Source: CAD feature listing. Evaluate the final solid. Frame: model axes, mm. A direction names the side the tool comes from. Coordinates: 2 decimals unless noted, no trailing zeros. Order: outer loops, then holes, each group sorted by start corner. A loop starts at its lowest first (then second) coordinate and runs counter-clockwise, first axis right, second up.
```python
from build123d import *

# Parameters (mm, degrees)
BOSS_EXTRUDE1_DEPTH = 15


with BuildPart() as part:
    # Sketch1 → Boss-Extrude1 (new body)
    with BuildSketch(Plane.XY):
        with BuildLine():
            Line((-3, 22.75), (-12, 16))
            ThreePointArc((-12, 16), (0, -20), (12, 16))
            Line((12, 16), (3, 22.75))
            ThreePointArc((3, 22.75), (0, 23.75), (-3, 22.75))
        make_face()
        with BuildLine():
            Line((2, 7.656854249), (-2, 7.656854249))
            Line((-2, 7.656854249), (-2, 5.656854249))
            ThreePointArc((-2, 5.656854249), (0, -6), (2, 5.656854249))
            Line((2, 5.656854249), (2, 7.656854249))
        make_face(mode=Mode.SUBTRACT)
    extrude(amount=BOSS_EXTRUDE1_DEPTH)


solid = part.part
```
1. Section query D-D, the plane x = -16. Output: boundary loops of the cut face in (y, z).
2. Section query A-A, the plane x = 0. Output: boundary loops of the cut face in (y, z).
3. Material intervals for line 1 along Y through (x, z) = (0, 7.25); line 2 along X through (y, z) = (0, 8); line 3 along X through (y, z) = (7.5, 6.25), sorted ascending.
4. Section query B-B, the plane y = 0. Output: boundary loops of the cut face in (x, z), plus the area to 3 significant figures.
5. Contact query for flat-ended pins moving along their axis: P1, Ø3, axis at x = 0, z = 7.5, coming from the -Y side; P2, Ø1.5, axis at x = -9.5, z = 4, coming from the +Y side; P3, Ø1.5, axis at x = -12.5, z = 12, coming from the -Y side. Output: stop coordinate, or through.
6. Access query for faces 1 (the flat face through (-2, 7, 7)), 2 (the flat face through (4, 7, 15)). Directions: +Z, -Z, +X, -X, +Y, -Y. A direction counts if a zero-diameter tool reaches every point of the face in a straight line with its end or side. Return the directions, or none.
7. Section query C-C, the plane z = 12. Output: boundary loops of the cut face in (x, y).
Answer key:
1. outline: (-12, 0) - (12, 0) - (12, 15) - (-12, 15) - close
2. outline: (-20, 0) - (-6, 0) - (-6, 15) - (-20, 15) - close; (7.66, 0) - (23.75, 0) - (23.75, 15) - (7.66, 15) - close
3. line 1: y = -20 to -6, 7.66 to 23.75
3. line 2: x = -20 to -6, 6 to 20
3. line 3: x = -18.54 to -2, 2 to 18.54
4. outline: (-20, 0) - (-6, 0) - (-6, 15) - (-20, 15) - close; (6, 0) - (20, 0) - (20, 15) - (6, 15) - close
4. area: 420 mm2
5. P1: stops at y = -20
5. P2: stops at y = 18.44
5. P3: stops at y = -16.18
6. face 1: +Z, -Z
6. face 2: +Z, +X, -X, +Y, -Y
7. outline: (-12, 16) arc R20 ccw (long way) to (12, 16) - (3, 22.75) arc R5 ccw to (-3, 22.75) - close; hole (-2, 5.66) arc R6 ccw (long way) to (2, 5.66) - (2, 7.66) - (-2, 7.66) - close
